```python
from build123d import *

# Parameters (mm, degrees)
F0_R     = 18.75028
F0_R_2   = 12.49934
F1_DEPTH = 99.9998
F3_DEPTH = 100.0008


with BuildPart() as f1:
    # F0 (on Top) → F1 (new body)
    with BuildSketch(Plane.XY):
        Circle(F0_R)
        Circle(F0_R_2, mode=Mode.SUBTRACT)
    extrude(amount=F1_DEPTH)

    # F2 (on face) → F3 (cut, through all)
    with BuildSketch(Plane.XY.offset(99.9998)):
        with BuildLine():
            ThreePointArc((-4.0005, 11.841854), (-7.288, -10.154731), (12.49934, 0))
            ThreePointArc((12.49934, 0), (10.154731, 7.288), (4.0005, 11.841854))
            Line((4.0005, 11.841854), (4.0005, 8.49884))
            Line((4.0005, 8.49884), (-4.0005, 8.49884))
            Line((-4.0005, 8.49884), (-4.0005, 11.841854))
        make_face()
        with BuildLine():
            ThreePointArc((-4.0005, 11.841854), (0, 12.49934), (4.0005, 11.841854))
            Line((4.0005, 11.841854), (4.0005, 16.49984))
            Line((4.0005, 16.49984), (-4.0005, 16.49984))
            Line((-4.0005, 16.49984), (-4.0005, 11.841854))
        make_face()
    extrude(amount=-F3_DEPTH, mode=Mode.SUBTRACT)


solid = f1.part
```
Can you work these out from the model? Positions are in its coordinate system, mm. A direction names the side the tool comes from. Coordinates: 2 decimals unless noted, no trailing zeros. Loops run counter-clockwise (first coordinate to the right, second up) from the corner with the lowest first, then second, coordinate; pieces in that order, holes last. Notation, with made-up numbers: M 6.25,-20.5 L 51.25,-20.5 A34 ccw 51.25,9.5 Z; hole C 55.25,28.5 d1. An arc over 180 degrees is marked long. Put each result on its own line as item: value. Start each with the question number.
(1) I need wall thicknesses on probe 1 along X at (y, z) = (-7.5, 13.5); probe 2 along X at (y, z) = (9.5, 45); probe 3 along Y at (x, z) = (3.5, 36.5). Which ranges of each line are inside material? Lowest first, please.
(2) Will these pins go through, and if not, where does the flat tip stop? pin 1 Ø1 at (y, z) = (13, 42.5) entering from +X; pin 2 Ø5 at (y, z) = (15, 58) entering from -X; pin 3 Ø1.5 at (x, z) = (11, 40) entering from -Y.
(3) Which directions (+Z, -Z, +X, -X, +Y, -Y) give clear straight access to the entire face, cutting with the end or side of a thin tool? Please do faces 1 (the face through (4, 14, 51)), 2 (the face through (3.9, -12.2, 100)).
(4) Imagine slicing it at A-A on y = 0. List the corners of the cut face in (x, z) for me, and give its area (3 significant figures).
(5) We'd pull the mould along X, two halves only. Please class faces 3 (the face through (3.9, -12.2, 0)), 4 (the face through (-14.88, -11.41, 49.3)), 5 (the face through (0, 16.5, 51)): +X half, -X half, draft (parallel to the pull), parting line (faces both ways), or undercut.
(6) Imagine slicing it at C-C on z = 70. List the corners of the cut face in (x, y) for me.
(7) Imagine slicing it at B-B on x = -10.5. List the corners of the cut face in (y, z) for me, and give its area (3 significant figures).
Worked answers:
1. probe 1: x = -17.18 to -10, 10 to 17.18
1. probe 2: x = -16.17 to -8.12, 8.12 to 16.17
1. probe 3: y = -18.42 to -12, 16.5 to 18.42
2. pin 1: stops at x = 13.98
2. pin 2: stops at x = -13.98
2. pin 3: stops at y = -15.7
3. face 1: +Z, -Z
3. face 2: +Z, +X, -X, +Y, -Y
4. outline: M -18.75,0 L -12.5,0 L -12.5,100 L -18.75,100 Z; M 12.5,0 L 18.75,0 L 18.75,100 L 12.5,100 Z
4. area: 1,250 mm2
5. face 3: draft
5. face 4: parting line
5. face 5: undercut
6. outline: C 0,0 d37.5; hole M -4,11.84 A12.5 ccw long 4,11.84 L 4,16.5 L -4,16.5 Z
7. outline: M -15.53,0 L -6.78,0 L -6.78,100 L -15.53,100 Z; M 6.78,0 L 15.53,0 L 15.53,100 L 6.78,100 Z
7. area: 1,750 mm2
